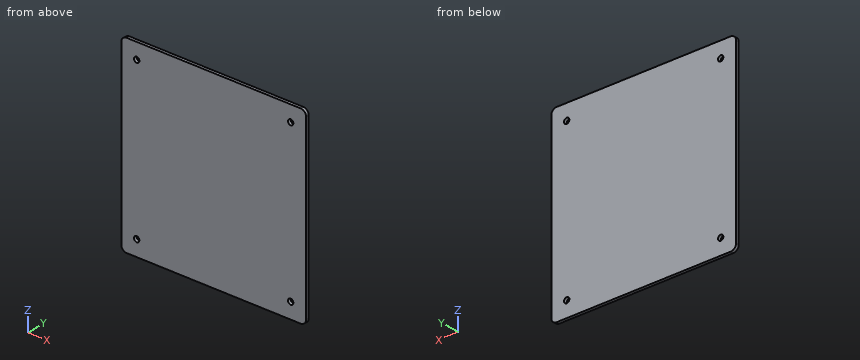
```python
from build123d import *

# Parameters (mm, degrees)
SKETCH_4_W          = 120
SKETCH_4_H          = 120
EXTRUDE_2_DEPTH     = 2
FILLET_2_R          = 3.5
SKETCH_5_R          = 1.75
CUT_EXTRUDE_1_DEPTH = 3


with BuildPart() as part:
    # 草图4 → 凸台-拉伸2 (new body)
    with BuildSketch(Plane(origin=(0, 0, 0), x_dir=(1, 0, 0), z_dir=(0, 1, 0))):
        Rectangle(SKETCH_4_W, SKETCH_4_H)
    extrude(amount=EXTRUDE_2_DEPTH)

    # 圆角2
    fillet_2_edges = [part.edges().sort_by_distance(p)[0] for p in [
        (60, 1, 60),
        (-60, 1, 60),
        (-60, 1, -60),
        (60, 1, -60),
    ]]
    fillet(fillet_2_edges, radius=FILLET_2_R)

    # 草图5 → 切除-拉伸1 (cut, through all)
    with BuildSketch(Plane(origin=(0, 2, 0), x_dir=(1, 0, 0), z_dir=(0, 1, 0))):
        with Locations((-50, 50)):
            Circle(SKETCH_5_R)
        with Locations((-50, -50)):
            Circle(SKETCH_5_R)
        with Locations((50, -50)):
            Circle(SKETCH_5_R)
        with Locations((50, 50)):
            Circle(SKETCH_5_R)
    extrude(amount=-CUT_EXTRUDE_1_DEPTH, mode=Mode.SUBTRACT)


solid = part.part
```
The listing builds one solid part. Answer for the finished solid, in the listing's coordinates (mm). Give positions to 0.01 mm unless a question says otherwise; leave off trailing zeros. Order: outer loops, then holes, each group sorted by start corner. A loop starts at its lowest first (then second) coordinate and runs counter-clockwise, first axis right, second up.
1) Find section B-B on z = -50. Write down the section's boundary in (x, y).
Reported:
outline: (-60, 0) - (-51.75, 0) - (-51.75, 2) - (-60, 2) - close; (-48.25, 0) - (48.25, 0) - (48.25, 2) - (-48.25, 2) - close; (51.75, 0) - (60, 0) - (60, 2) - (51.75, 2) - close
2) Find section A-A on x = 50. Write down the section's boundary in (y, z).
Reported:
outline: (0, -60) - (2, -60) - (2, -51.75) - (0, -51.75) - close; (0, -48.25) - (2, -48.25) - (2, 48.25) - (0, 48.25) - close; (0, 51.75) - (2, 51.75) - (2, 60) - (0, 60) - close
3) Consider line 1 along X through (y, z) = (0.5, 50); line 2 along X through (y, z) = (0.15, -49). Determine where each line is inside the solid, lowest interval first.
Reported:
line 1: x = -60 to -51.75, -48.25 to 48.25, 51.75 to 60
line 2: x = -60 to -51.44, -48.56 to 48.56, 51.44 to 60
